```python
from build123d import *

# Parameters (mm, degrees)
BOSS_EXTRUDE2_DEPTH   = 8
M3_TAPPED_HOLE1_D     = 2.5
M3_TAPPED_HOLE1_DEPTH = 8.5
M3_TAPPED_HOLE1_TIP   = 0.751075774
M4_TAPPED_HOLE1_D     = 3.3
M4_TAPPED_HOLE1_DEPTH = 11.5
M4_TAPPED_HOLE1_TIP   = 0.991420021


with BuildPart() as part:
    # Sketch1 → Boss-Extrude2 (new body)
    with BuildSketch(Plane(origin=(0, 0, 0), x_dir=(1, 0, 0), z_dir=(0, 1, 0))):
        Polygon((35.397046685, 0.212206196), (35.397046685, -3.787793804), (-2.283249607, -3.787793804), (-2.283249607, -8.787793804), (-9.783249607, -8.787793804), (-18.892613672, -6.346947059), (-28.102933344, -8.814844777), (-34.602933344, -8.814844777), (-34.602933344, -4.117707659), (-27.103302555, 0.212206196), align=None)
    extrude(amount=BOSS_EXTRUDE2_DEPTH)

    # M3 Tapped Hole1
    with Locations(Plane(origin=(0, 0, -0.212206196), x_dir=(-1, 0, 0), z_dir=(0, 0, -1))):
        with Locations((-31.397046685, 4), (-24.397046685, 4)):
            Hole(M3_TAPPED_HOLE1_D / 2, depth=M3_TAPPED_HOLE1_DEPTH)
            with Locations((0, 0, -(M3_TAPPED_HOLE1_DEPTH + M3_TAPPED_HOLE1_TIP / 2))):  # 118° drill point
                Cone(0, M3_TAPPED_HOLE1_D / 2, M3_TAPPED_HOLE1_TIP, mode=Mode.SUBTRACT)

    # M4 Tapped Hole1
    with Locations(Plane(origin=(0, 0, -0.212206196), x_dir=(-1, 0, 0), z_dir=(0, 0, -1))):
        with Locations((18.892933344, 4)):
            Hole(M4_TAPPED_HOLE1_D / 2, depth=M4_TAPPED_HOLE1_DEPTH)
            with Locations((0, 0, -(M4_TAPPED_HOLE1_DEPTH + M4_TAPPED_HOLE1_TIP / 2))):  # 118° drill point
                Cone(0, M4_TAPPED_HOLE1_D / 2, M4_TAPPED_HOLE1_TIP, mode=Mode.SUBTRACT)


solid = part.part
```
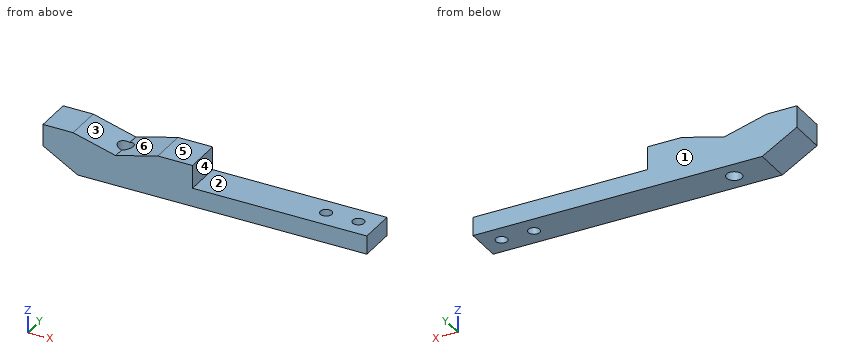
Check sheet for the modelled part. Datum: model origin and axes. Units: mm. Face numbers are marked on the shaded views. A direction names the side the tool comes from. Coordinates: 2 decimals unless noted, no trailing zeros. Order: outer loops, then holes, each group sorted by start corner. A loop starts at its lowest first (then second) coordinate and runs counter-clockwise, first axis right, second up. Notation, with made-up numbers: (9.5, 75) -> (22.5, 75) arc R19 cw to (22.5, 103) -> close; hole circle Ø4 at (-12.5, -22). An arc over 180 degrees is marked (long way). Write each question's results on one line, items separated by ' | '. Start each with the question number.
1) Section check A-A (z = 7.75). Enter the section's corners in (x, y).
2) Section check C-C (z = 5). Enter the section's corners in (x, y).
3) Section check D-D (x = 29). Enter the section's corners in (y, z), and give its area (3 significant figures).
4) Set-up check for the marked faces 1, 2 and 3: record each of +Z, -Z, +X, -X, +Y, -Y from which the full face is reachable in a straight line by a thin tool's end or side.
5) Draft check along X on the marked faces 4, 5 and 6. Enter one of: pulls with the +X half, pulls with the -X half, needs draft (parallel to the pull), parting line crosses it, or undercut.
6) Material ranges on line 1 along X through (y, z) = (4, 5); line 2 along X through (y, z) = (4.25, 3.75); line 3 along X through (y, z) = (3.75, 1.25), recorded low to high.
7) Depth check by flat-ended pin: pin 1 (1 mm diameter, centred on x = 8, y = 2, fed in from +Z); pin 2 (4.5 mm diameter, centred on x = -18.89, y = 4, fed in from +Z); pin 3 (4 mm diameter, centred on y = 5.5, z = 7, fed in from +X). Enter the tip coordinate at first touch or a pass-through.
8) Section check B-B (y = 4). Enter the section's corners in (x, z).
Checked values:
1) outline: (-34.6, 0) -> (-24.13, 0) -> (-24.13, 8) -> (-34.6, 8) -> close; (-13.66, 0) -> (-2.28, 0) -> (-2.28, 8) -> (-13.66, 8) -> close
2) outline: (-34.6, 0) -> (-2.28, 0) -> (-2.28, 8) -> (-34.6, 8) -> close; hole circle Ø3.3 at (-18.89, 4)
3) outline: (0, -0.21) -> (8, -0.21) -> (8, 3.79) -> (0, 3.79) -> close | area: 32.0 mm²
4) face 1: +Z, -Z, +X, -X, +Y | face 2: +Z, +X, +Y, -Y | face 3: +Z, +Y, -Y
5) face 4: pulls with the +X half | face 5: needs draft | face 6: undercut
6) line 1: -34.6 to -20.54, -17.24 to -2.28 | line 2: -33.97 to -20.52, -17.26 to 23.17, 25.62 to 30.17, 32.62 to 35.4 | line 3: -29.64 to -20.52, -17.26 to 23.17, 25.62 to 30.17, 32.62 to 35.4
7) pin 1: z = 3.79 | pin 2: z = 6.95 | pin 3: x = -2.28
8) outline: (-34.6, 4.12) -> (-27.1, -0.21) -> (-20.54, -0.21) -> (-20.54, 6.79) -> (-28.1, 8.81) -> (-34.6, 8.81) -> close; (-17.24, -0.21) -> (23.15, -0.21) -> (23.15, 3.79) -> (-2.28, 3.79) -> (-2.28, 8.79) -> (-9.78, 8.79) -> (-17.24, 6.79) -> close; (25.65, -0.21) -> (30.15, -0.21) -> (30.15, 3.79) -> (25.65, 3.79) -> close; (32.65, -0.21) -> (35.4, -0.21) -> (35.4, 3.79) -> (32.65, 3.79) -> close
